The listing builds one solid part. Answer for the finished solid, in the listing's coordinates (mm). A direction names the side the tool comes from. Coordinates: 2 decimals unless noted, no trailing zeros. Write item = value, one per line. Start each with the question number.
```python
from build123d import *

# Parameters (mm, degrees)
SKETCH1_R           = 6.35
BOSS_EXTRUDE1_DEPTH = 5.08
FILLET1_R           = 1.27
BOSS_EXTRUDE2_DEPTH = 2.54
CHAMFER1_SIZE       = 3.81
CHAMFER1_SIZE_2     = 1.776632178
FILLET2_R           = 25.4


with BuildPart() as part:
    # Sketch1 → Boss-Extrude1 (new, symmetric)
    with BuildSketch(Plane(origin=(0, 0, 0), x_dir=(0, 0, -1), z_dir=(1, 0, 0))):
        with BuildLine():
            Line((-88.177460957, -43.18), (-95.797460957, -27.94))
            Line((-95.797460957, -27.94), (-19.494713075, -10.16))
            ThreePointArc((-19.494713075, -10.16), (-13.691248965, -6.485853779), (-11.43, 0))
            ThreePointArc((-11.43, 0), (2.608865683, 11.128284677), (10.23906734, -5.08))
            ThreePointArc((10.23906734, -5.08), (7.261735691, -17.78), (10.23906734, -30.48))
            ThreePointArc((10.23906734, -30.48), (9.389887981, -39.759205985), (0.722539043, -43.18))
            ThreePointArc((0.722539043, -43.18), (-43.727460957, -39.260382077), (-88.177460957, -43.18))
        make_face()
        Circle(SKETCH1_R, mode=Mode.SUBTRACT)
    extrude(amount=BOSS_EXTRUDE1_DEPTH, both=True)

    # Fillet1
    fillet1_edges = [part.edges().sort_by_distance(p)[0] for p in [
        (5.08, -39.260382077, 43.727460957),
        (5.08, -39.759205985, -9.389887981),
        (5.08, -17.78, -7.261735691),
        (5.08, 11.128284677, -2.608865683),
        (5.08, -6.485853779, 13.691248965),
        (-5.08, 11.128284677, -2.608865683),
        (5.08, -19.05, 57.646087016),
        (-5.08, -17.78, -7.261735691),
        (-5.08, -39.759205985, -9.389887981),
        (-5.08, -39.260382077, 43.727460957),
        (-5.08, -19.05, 57.646087016),
        (-5.08, -6.485853779, 13.691248965),
    ]]
    fillet(fillet1_edges, radius=FILLET1_R)

    # Sketch3 → Boss-Extrude2 (add, symmetric)
    with BuildSketch(Plane(origin=(0, 0, 0), x_dir=(0, 0, -1), z_dir=(1, 0, 0))):
        Polygon((-93.892460957, -31.75), (-106.592460957, -34.925), (-112.942460957, -43.18), (-92.622460957, -42.339662192), (-43.915351624, -37.990451226), align=None)
    extrude(amount=BOSS_EXTRUDE2_DEPTH, both=True)

    # Chamfer1
    # the kernel refuses this chamfer: 3.81, 1.776632178 mm, written as the material it takes off along each edge
    with BuildSketch(Plane(origin=(-2.54, -43.587894094, 122.805646834), x_dir=(-0.016311164131110324, 0.9990130464553615, 0.041314391398951954), z_dir=(0, 0.041319888426956664, -0.999145968725483))) as chamfer1_piece_1_section:
        Polygon((CHAMFER1_SIZE * 0.999866964113, CHAMFER1_SIZE * 0.0163111641311), (-CHAMFER1_SIZE_2 * 0.0163111641272, CHAMFER1_SIZE_2 * 0.999866963871), (0, 0), align=None)
    chamfer1_piece_1 = extrude(amount=40.080601841, mode=Mode.PRIVATE)
    chamfer1_piece_1 = split(chamfer1_piece_1, bisect_by=Plane(origin=(-1.976451392, -34.769993735, 92.38246409), z_dir=(0, -0.44721359549995887, 0.8944271909999154)), keep=Keep.TOP, mode=Mode.PRIVATE)
    add(chamfer1_piece_1, mode=Mode.SUBTRACT)
    with BuildSketch(Plane(origin=(2.54, -43.587894094, 122.805646834), x_dir=(0.016311164131110324, 0.9990130464553615, 0.041314391398951954), z_dir=(0, 0.041319888426956664, -0.999145968725483))) as chamfer1_piece_2_section:
        Polygon((CHAMFER1_SIZE * 0.999866964113, -CHAMFER1_SIZE * 0.0163111641311), (-CHAMFER1_SIZE_2 * 0.0163111641272, -CHAMFER1_SIZE_2 * 0.999866963871), (0, 0), align=None)
    chamfer1_piece_2 = extrude(amount=40.080601841, mode=Mode.PRIVATE)
    chamfer1_piece_2 = split(chamfer1_piece_2, bisect_by=Plane(origin=(1.976451392, -34.769993735, 92.38246409), z_dir=(0, -0.44721359549995887, 0.8944271909999154)), keep=Keep.TOP, mode=Mode.PRIVATE)
    add(chamfer1_piece_2, mode=Mode.SUBTRACT)

    # Fillet2
    fillet2_edges = [part.edges().sort_by_distance(p)[0] for p in [
        (0, -34.925, 106.592460957),
    ]]
    fillet(fillet2_edges, radius=FILLET2_R)

    # Chamfer2
    # the kernel refuses this chamfer: 1.27, 0.83499617 mm, written as the material it takes off along each edge
    with BuildSketch(Plane(origin=(-0.763367822, -43.506315275, 120.833009659), x_dir=(0.9993026620124814, -0.03730696112582517, -0.0015428371024072082), z_dir=(0, 0.04131988842701986, -0.9991459687254804))) as chamfer2_piece_1_section:
        with BuildLine():
            Line((0.874521065, 0), (-0.619435505, -1.161345341))
            Line((-0.619435505, -1.161345341), (-0.642038856, -1.149758774))
            ThreePointArc((-0.642038856, -1.149758774), (-0.322768515, -0.573982799), (-0.022603351, 0.011586567))
            Line((-0.022603351, 0.011586567), (0.000948407, 0.025382288))
            ThreePointArc((0.000948407, 0.025382288), (0.437599315, 0.009066868), (0.875469472, 0.025382288))
            Line((0.875469472, 0.025382288), (0.874521065, 0))
        make_face()
    chamfer2_piece_1 = extrude(amount=36.131955223, mode=Mode.PRIVATE)
    chamfer2_piece_1 = split(chamfer2_piece_1, bisect_by=Plane(origin=(-0.672553729, -35.934823141, 91.800049387), z_dir=(0, -0.44721359549995887, 0.8944271909999154)), keep=Keep.TOP, mode=Mode.PRIVATE)
    add(chamfer2_piece_1, mode=Mode.SUBTRACT)
    with BuildSketch(Plane(origin=(0.763367822, -43.506315275, 120.833009659), x_dir=(0.4373449734128742, 0.8985257946973667, 0.03715872029494756), z_dir=(0, 0.04131988842701986, -0.9991459687254804))) as chamfer2_piece_2_section:
        with BuildLine():
            Line((1.316215539, 0), (-0.411565873, -0.771622074))
            Line((-0.411565873, -0.771622074), (-0.434407936, -0.760513512))
            ThreePointArc((-0.434407936, -0.760513512), (-0.213942404, -0.381842921), (-0.022842063, 0.011108562))
            Line((-0.022842063, 0.011108562), (0.000414304, 0.025396621))
            ThreePointArc((0.000414304, 0.025396621), (0.658346981, 0.014663545), (1.316629843, 0.025396621))
            Line((1.316629843, 0.025396621), (1.316215539, 0))
        make_face()
    chamfer2_piece_2 = extrude(amount=36.131955223, mode=Mode.PRIVATE)
    chamfer2_piece_2 = split(chamfer2_piece_2, bisect_by=Plane(origin=(0.672553729, -35.934823141, 91.800049387), z_dir=(0, -0.44721359549995887, 0.8944271909999154)), keep=Keep.TOP, mode=Mode.PRIVATE)
    add(chamfer2_piece_2, mode=Mode.SUBTRACT)


solid = part.part
```
1. Each of these flat-tipped pins is pushed along its axis until it touches: pin 1 (3.5 mm diameter, centred on y = -33.5, z = 97, fed in from -X); pin 2 (3.5 mm diameter, centred on y = -35, z = 98.5, fed in from +X); pin 3 (1.5 mm diameter, centred on x = 3, y = -12.5, fed in from -Z); pin 4 (14.5 mm diameter, centred on y = 0, z = 0, fed in from +X). Where does it stop, or does it pass through?
2. For a pull along Y with two mould halves and no side action, classify faces 4 (the face through (-0.07, -6.2, 1.38)), 5 (the face through (0.05, -6.56, 13.75)), 6 (the face through (-2.54, -36, 98)) as pulls with the +Y half, pulls with the -Y half, needs draft (parallel to the pull), parting line crosses it, or undercut.
3. Straight lines are drawn through the part: L1, parallel to Y at x = -2.75, z = 0; L2, parallel to Z at x = 0.5, y = 5.5; L3, parallel to Y at x = 4, z = 78. For each, find the intervals that lie inside material, in ascending order. Write a range as [from, to].
4. For faces 1 (the face through (0.036, -32.258, 95.924)), 2 (the face through (2.54, -36, 98)), 3 (the face through (0.053, -19.174, 58.18)), determine the directions among +Z, -Z, +X, -X, +Y, -Y from which every point of the face is accessible in a straight line to the end or side of a thin tool.
Solution:
q1.pin_1 = -2.54
q1.pin_2 = 2.54
q1.pin_3 = -7.91
q1.pin_4 = 5.08
q2.face_4 = undercut
q2.face_5 = pulls with the +Y half
q2.face_6 = needs draft
q3.L1 = [-43.05, -6.35], [6.35, 11.43]
q3.L2 = [-10.02, -3.17], [3.17, 10.02]
q3.L3 = [-41.57, -23.81]
q4.face_1 = +Z, +X, -X
q4.face_2 = +Z, +X, -Y
q4.face_3 = +Z, +X, -X, +Y
